from build123d import *

# Parameters (mm, degrees)
F0_W      = 280
F0_H      = 110
F1_DEPTH  = 8
F2_W      = 280
F2_H      = 110
F2_W_2    = 264
F2_H_2    = 94
F3_DEPTH  = 20
F5_DEPTH  = 340
F6_W      = 224
F6_H      = 8
F7_DEPTH  = 20
F8_W      = 280
F8_H      = 110
F8_W_2    = 264
F8_H_2    = 94
F9_DEPTH  = 8
F10_R     = 1.55
F11_DEPTH = 8
F12_W     = 220
F12_H     = 30
F13_DEPTH = 8
F14_R     = 5


# Not quite as in the source:
# - a feature names something its author has since deleted; it is built from what else it names


with BuildPart() as f1:
    # F0 (on Top) → F1 (new body)
    with BuildSketch(Plane.XY):
        Rectangle(F0_W, F0_H)
    extrude(amount=F1_DEPTH)

    # F2 (on face) → F3 (join)
    with BuildSketch(Plane.XY.offset(8)):
        Rectangle(F2_W, F2_H)
        Rectangle(F2_W_2, F2_H_2, mode=Mode.SUBTRACT)
    extrude(amount=F3_DEPTH)

    # F4 (on face) → F5 (join)
    with BuildSketch(Plane.XY.offset(28)):
        Polygon((-132, -47), (-132, 47), (132, 47), (132, -47), (112, -47), (112, -55), (140, -55), (140, 55), (-140, 55), (-140, -55), (-112, -55), (-112, -47), align=None)
    extrude(amount=F5_DEPTH)

    # F6 (on face) → F7 (join)
    with BuildSketch(Plane.XY.offset(368)):
        Polygon((-112, -47), (-132, -47), (-132, 47), (132, 47), (132, -47), (112, -47), (112, -55), (140, -55), (140, 55), (-140, 55), (-140, -55), (-112, -55), align=None)
        with Locations((0, -51)):
            Rectangle(F6_W, F6_H)
    extrude(amount=F7_DEPTH)

    # F8 (on face) → F9 (join)
    with BuildSketch(Plane.XY.offset(388)):
        Rectangle(F8_W, F8_H)
        Rectangle(F8_W_2, F8_H_2, mode=Mode.SUBTRACT)
        Rectangle(F8_W_2, F8_H_2)
    extrude(amount=F9_DEPTH)

    # F10 (on face) → F11 (cut, through all)
    with BuildSketch(Plane.YZ.offset(140)):
        with Locations((0, 80)):
            Circle(F10_R)
        with Locations((0, 70)):
            Circle(F10_R)
        with Locations((0, 50)):
            Circle(F10_R)
        with Locations((0, 40)):
            Circle(F10_R)
        with Locations((0, 60)):
            Circle(F10_R)
    extrude(amount=-F11_DEPTH, mode=Mode.SUBTRACT)

    # F12 (on face) → F13 (cut, through all)
    with BuildSketch(Plane.XY.offset(396)):
        Rectangle(F12_W, F12_H)
    extrude(amount=-F13_DEPTH, mode=Mode.SUBTRACT)

    # F14
    f14_edges = [f1.edges().sort_by_distance(p)[0] for p in [
        (-110, 15, 392),
        (-110, -15, 392),
        (110, -15, 392),
        (110, 15, 392),
    ]]
    fillet(f14_edges, radius=F14_R)


solid = f1.part
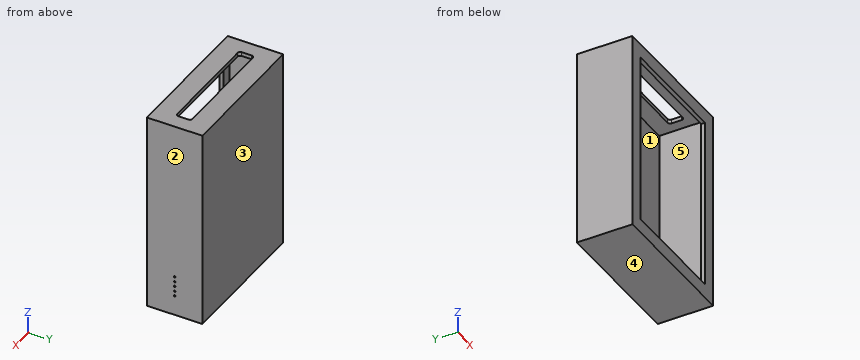
Could you check a few things on this model? Use its own coordinates, in mm. Face numbers are marked on the shaded views. A direction names the side the tool comes from. Coordinates: 2 decimals unless noted, no trailing zeros. Write each loop counter-clockwise with the first axis right and the second up, starting at its lowest first coordinate (ties: lowest second). Pieces come first, ordered by that corner, then holes. Notation, with made-up numbers: (-1.75, 73.25) - (38.25, 73.25) arc R16 ccw to (38.25, 97.25) - close; hole circle Ø4 at (28, -14.5). An arc over 180 degrees is marked (long way). Put each result on its own line as item: value. Start each with the question number.
Q1. I want a section at C-C on z = 312.5. Write out the boundary of the cut face in (x, y).
Q2. Which directions (+Z, -Z, +X, -X, +Y, -Y) give clear straight access to the entire face, cutting with the end or side of a thin tool? Please do the marked faces 1 and 2.
Q3. Thinking about a two-plate mould opening in Z: for the marked faces 3, 4 and 5, which applies, pulls with the +Z half, pulls with the -Z half, needs draft (parallel to the pull), parting line crosses it, or undercut?
Q4. I want a section at A-A on x = -100. Write out the boundary of the cut face in (y, z), plus the area to 3 significant figures.
Q5. Please list where these lines run through material, in increasing order: L1, parallel to Z at x = 134.75, y = 0; L2, parallel to Y at x = 123, z = 205.5; L3, parallel to Z at x = -41, y = 43.
Q6. I want a section at B-B on x = 120.5. Write out the boundary of the cut face in (y, z), plus the area to 3 significant figures.
Q7. I'm going to push flat-ended pins straight in: P1, Ø5, axis at x = -47, y = -11, coming from the +Z side; P2, Ø2, axis at x = 0.5, z = 283.5, coming from the -Y side; P3, Ø3, axis at y = 0, z = 70, coming from the +X side. Where does each tip first touch, or does it pass through?
Checks:
1. outline: (-140, -55) - (-112, -55) - (-112, -47) - (-132, -47) - (-132, 47) - (132, 47) - (132, -47) - (112, -47) - (112, -55) - (140, -55) - (140, 55) - (-140, 55) - close
2. face 1: none
2. face 2: +Z, -Z, +X, +Y, -Y
3. face 3: needs draft
3. face 4: pulls with the -Z half
3. face 5: undercut
4. outline: (-55, 0) - (55, 0) - (55, 396) - (15, 396) - (15, 388) - (47, 388) - (47, 8) - (-47, 8) - (-47, 28) - (-55, 28) - close; (-55, 368) - (-47, 368) - (-47, 388) - (-15, 388) - (-15, 396) - (-55, 396) - close
4. area: 4,880 mm²
5. L1: 0 to 38.45, 41.55 to 48.45, 51.55 to 58.45, 61.55 to 68.45, 71.55 to 78.45, 81.55 to 396
5. L2: -55 to -47, 47 to 55
5. L3: 0 to 8, 388 to 396
6. outline: (-55, 0) - (55, 0) - (55, 396) - (-55, 396) - close; hole (-47, 8) - (47, 8) - (47, 388) - (-47, 388) - close
6. area: 7,840 mm²
7. P1: z = 8
7. P2: y = 47
7. P3: x = -132
